from build123d import *

# Parameters (mm, degrees)
SKETCH_W        = 50
SKETCH_H        = 35
PAD_DEPTH       = 3
SKETCH002_W     = 45
SKETCH002_H     = 30
PAD001_DEPTH    = 1.5
SKETCH003_W     = 43
SKETCH003_H     = 28
POCKET001_DEPTH = 2.5
FILLET_R        = 1
FILLET001_R     = 1
SKETCH005_R     = 2.5
PAD002_DEPTH    = 5
SKETCH004_R     = 2.5
PAD003_DEPTH    = 5
SKETCH006_R     = 1.75
POCKET_DEPTH    = 5
SKETCH007_R     = 1.75
POCKET002_DEPTH = 5
CHAMFER_SIZE    = 1.5
CHAMFER001_SIZE = 1.5


with BuildPart() as part:
    # Sketch → Pad (new body)
    with BuildSketch(Plane.XY):
        Rectangle(SKETCH_W, SKETCH_H)
    extrude(amount=PAD_DEPTH)

    # Sketch002 → Pad001 (join)
    with BuildSketch(Plane.XY.offset(3)):
        Rectangle(SKETCH002_W, SKETCH002_H)
    extrude(amount=PAD001_DEPTH)

    # Sketch003 (on Face11 of Pad001) → Pocket001 (cut)
    with BuildSketch(Plane.XY.offset(4.5)):
        Rectangle(SKETCH003_W, SKETCH003_H)
    extrude(amount=-POCKET001_DEPTH, mode=Mode.SUBTRACT)

    # Fillet
    fillet_edges = [part.edges().sort_by_distance(p)[0] for p in [
        (0, 17.5, 0),
        (-25, 17.5, 1.5),
        (-25, 0, 0),
        (-25, -17.5, 1.5),
        (0, -17.5, 0),
        (25, -17.5, 1.5),
        (25, 0, 0),
        (25, 17.5, 1.5),
    ]]
    fillet(fillet_edges, radius=FILLET_R)

    # Fillet001
    fillet001_edges = [part.edges().sort_by_distance(p)[0] for p in [
        (-21.5, -14, 3.25),
        (22.5, -15, 3.75),
        (22.5, 15, 3.75),
        (-22.5, 15, 3.75),
        (-22.5, -15, 3.75),
        (21.5, 14, 3.25),
        (-21.5, 14, 3.25),
        (21.5, -14, 3.25),
    ]]
    fillet(fillet001_edges, radius=FILLET001_R)

    # Sketch005 → Pad002 (join)
    with BuildSketch(Plane.XY):
        with Locations((-19.25, 11.75)):
            Circle(SKETCH005_R)
    extrude(amount=PAD002_DEPTH)

    # Sketch004 (on Face35 of Fillet001) → Pad003 (join)
    with BuildSketch(Plane(origin=(0, 0, 0), x_dir=(1, 0, 0), z_dir=(0, 0, -1))):
        with Locations((19.25, 11.75)):
            Circle(SKETCH004_R)
    extrude(amount=-PAD003_DEPTH)

    # Sketch006 (on Face48 of Pad003) → Pocket (cut)
    with BuildSketch(Plane(origin=(0, 0, 0), x_dir=(1, 0, 0), z_dir=(0, 0, -1))):
        with Locations((-19.25, -11.75)):
            Circle(SKETCH006_R)
    extrude(amount=-POCKET_DEPTH, mode=Mode.SUBTRACT)

    # Sketch007 (on Face48 of Pocket) → Pocket002 (cut)
    with BuildSketch(Plane(origin=(0, 0, 0), x_dir=(1, 0, 0), z_dir=(0, 0, -1))):
        with Locations((19.25, 11.75)):
            Circle(SKETCH007_R)
    extrude(amount=-POCKET002_DEPTH, mode=Mode.SUBTRACT)

    # Chamfer
    chamfer_edges = [part.edges().sort_by_distance(p)[0] for p in [
        (-21, 11.75, 0),
    ]]
    chamfer(chamfer_edges, length=CHAMFER_SIZE)

    # Chamfer001
    chamfer001_edges = [part.edges().sort_by_distance(p)[0] for p in [
        (17.5, -11.75, 0),
    ]]
    chamfer(chamfer001_edges, length=CHAMFER001_SIZE)


solid = part.part
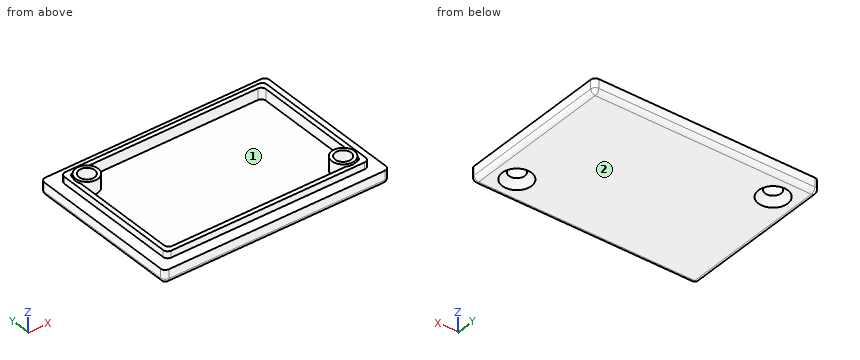
The listing builds one solid part. Answer for the finished solid, in the listing's coordinates (mm). Face numbers are marked on the shaded views. Round coordinates to 2 decimals unless told otherwise and drop trailing zeros. Write each loop counter-clockwise with the first axis right and the second up, starting at its lowest first coordinate (ties: lowest second). Pieces come first, ordered by that corner, then holes. Notation, with made-up numbers: (12, 8) - (56, 8) arc R12 cw to (56, 26) - close; hole circle Ø9 at (54, 18). An arc over 180 degrees is marked (long way). Use one line per item in the form item = value. Start each with the question number.
Item 1: A cutting plane is placed at B-B (y = -11.75). Write down the section's boundary in (x, z), plus the area to 3 significant figures.
Item 2: Flat-ended cylindrical pins translate along their axes: pin 1 Ø8 at (x, y) = (-15, 3.5) entering from +Z; pin 2 Ø1.5 at (y, z) = (5.5, 4) entering from +X; pin 3 Ø2 at (x, y) = (19.25, -11.75) entering from +Z; pin 4 Ø1.6 at (x, z) = (-8, 4) entering from +Y. Find the tip coordinate at first contact, or state that the pin passes through.
Item 3: Find the intervals of material crossed by line 1 (Y direction, x = -19.25, z = 2.8); line 2 (X direction, y = 11.75, z = 2.8); line 3 (Y direction, x = 19.25, z = 3.5), in increasing order. Write a range as [from, to].
Item 4: A cutting plane is placed at D-D (x = -2.5). Write down the section's boundary in (y, z).
Item 5: Determine the mould class of the marked faces 1 and 2 for opening direction X: +X half, -X half, draft (parallel to the pull), parting line (faces both ways), or undercut.
Item 6: A cutting plane is placed at A-A (x = -19.25). Write down the section's boundary in (y, z), plus the area to 3 significant figures.
Item 7: A cutting plane is placed at C-C (z = 3.5). Write down the section's boundary in (x, y).
The answers:
q1.outline = (-25, 1) arc R1 ccw to (-24, 0) - (16, 0) - (17.5, 1.5) - (17.5, 5) - (16.75, 5) - (16.75, 2) - (-21.5, 2) - (-21.5, 4.5) - (-22.5, 4.5) - (-22.5, 3) - (-25, 3) - close; (21, 1.5) - (22.5, 0) - (24, 0) arc R1 ccw to (25, 1) - (25, 3) - (22.5, 3) - (22.5, 4.5) - (21.75, 4.5) - (21.75, 5) - (21, 5) - close
q1.area = 104 mm^2
q2.pin_1 = 2
q2.pin_2 = 22.5
q2.pin_3 = through
q2.pin_4 = 15
q3.line_1 = [-17.5, -14], [9.25, 10], [13.5, 17.5]
q3.line_2 = [-25, -21], [-17.5, -16.75], [21.5, 25]
q3.line_3 = [-15, -13.5], [-10, -9.25], [14, 15]
q4.outline = (-17.5, 1) arc R1 ccw to (-16.5, 0) - (16.5, 0) arc R1 ccw to (17.5, 1) - (17.5, 3) - (15, 3) - (15, 4.5) - (14, 4.5) - (14, 2) - (-14, 2) - (-14, 4.5) - (-15, 4.5) - (-15, 3) - (-17.5, 3) - close
q5.face_1 = undercut
q5.face_2 = draft
q6.outline = (-17.5, 1) arc R1 ccw to (-16.5, 0) - (8.5, 0) - (10, 1.5) - (10, 5) - (9.25, 5) - (9.25, 2) - (-14, 2) - (-14, 4.5) - (-15, 4.5) - (-15, 3) - (-17.5, 3) - close; (13.5, 1.5) - (15, 0) - (16.5, 0) arc R1 ccw to (17.5, 1) - (17.5, 3) - (15, 3) - (15, 4.5) - (14.25, 4.5) - (14.25, 5) - (13.5, 5) - close
q6.area = 74.2 mm^2
q7.outline = (-22.5, -14) arc R1 ccw to (-21.5, -15) - (21.5, -15) arc R1 ccw to (22.5, -14) - (22.5, 14) arc R1 ccw to (21.5, 15) - (-21.5, 15) arc R1 ccw to (-22.5, 14) - close; hole (-21.5, -13) arc R1 ccw to (-20.5, -14) - (18.16, -14) arc R2.5 cw (long way) to (21.5, -10.66) - (21.5, 13) arc R1 ccw to (20.5, 14) - (-18.16, 14) arc R2.5 cw (long way) to (-21.5, 10.66) - close; hole (-21.5, 12.84) arc R2.5 cw to (-20.34, 14) - (-20.5, 14) arc R1 ccw to (-21.5, 13) - close; hole circle Ø3.5 at (-19.25, 11.75); hole circle Ø3.5 at (19.25, -11.75); hole (20.34, -14) - (20.5, -14) arc R1 ccw to (21.5, -13) - (21.5, -12.84) arc R2.5 cw to start
